from build123d import *

# Parameters (mm, degrees)
SKETCH1_R                      = 5.5
BOSS_EXTRUDE1_DEPTH            = 5
BOSS_EXTRUDE2_DEPTH            = 2
SKETCH4_R                      = 1.4
BOSS_EXTRUDE3_DEPTH            = 7
SKETCH12_W                     = 20
SKETCH12_H                     = 2
CUT_EXTRUDE1_DEPTH             = 10
F_4_2_4_2_DIAMETER_HOLE1_D     = 4.2
F_4_2_4_2_DIAMETER_HOLE1_DEPTH = 20
F_4_2_4_2_DIAMETER_HOLE1_TIP   = 1.2618073
F_5_0_5_DIAMETER_HOLE1_D       = 5
F_5_0_5_DIAMETER_HOLE1_DEPTH   = 5
F_5_0_5_DIAMETER_HOLE1_TIP     = 1.502151548


with BuildPart() as part:
    # Sketch1 → Boss-Extrude1 (new body)
    with BuildSketch(Plane(origin=(0, 111.722415865, 0), x_dir=(1, 0, 0), z_dir=(0, 1, 0))):
        with BuildLine():
            Line((241.95107426, 942.218289838), (411.95107426, 942.218289838))
            ThreePointArc((411.95107426, 942.218289838), (419.022142072, 945.147222026), (421.95107426, 952.218289838))
            Line((421.95107426, 952.218289838), (421.95107426, 1052.218289838))
            ThreePointArc((421.95107426, 1052.218289838), (419.022142072, 1059.28935765), (411.95107426, 1062.218289838))
            Line((411.95107426, 1062.218289838), (241.95107426, 1062.218289838))
            ThreePointArc((241.95107426, 1062.218289838), (234.880006448, 1059.28935765), (231.95107426, 1052.218289838))
            Line((231.95107426, 1052.218289838), (231.95107426, 952.218289838))
            ThreePointArc((231.95107426, 952.218289838), (234.880006448, 945.147222026), (241.95107426, 942.218289838))
        make_face()
        with Locations(Location((241.95107426, 952.218289838, 0), (0, 0, 270))):
            Circle(SKETCH1_R, mode=Mode.SUBTRACT)
        with Locations(Location((411.95107426, 952.218289838, 0), (0, 0, 270))):
            Circle(SKETCH1_R, mode=Mode.SUBTRACT)
        with Locations(Location((411.95107426, 1052.218289838, 0), (0, 0, 270))):
            Circle(SKETCH1_R, mode=Mode.SUBTRACT)
        with Locations(Location((241.95107426, 1052.218289838, 0), (0, 0, 270))):
            Circle(SKETCH1_R, mode=Mode.SUBTRACT)
        with BuildLine():
            Line((249.45107426, 952.218289838), (249.45107426, 944.718289838))
            Line((249.45107426, 944.718289838), (404.45107426, 944.718289838))
            Line((404.45107426, 944.718289838), (404.45107426, 952.218289838))
            ThreePointArc((404.45107426, 952.218289838), (406.647773401, 957.521590697), (411.95107426, 959.718289838))
            Line((411.95107426, 959.718289838), (419.45107426, 959.718289838))
            Line((419.45107426, 959.718289838), (419.45107426, 1044.718289838))
            Line((419.45107426, 1044.718289838), (411.95107426, 1044.718289838))
            ThreePointArc((411.95107426, 1044.718289838), (406.647773401, 1046.914988979), (404.45107426, 1052.218289838))
            Line((404.45107426, 1052.218289838), (404.45107426, 1059.718289838))
            Line((404.45107426, 1059.718289838), (249.45107426, 1059.718289838))
            Line((249.45107426, 1059.718289838), (249.45107426, 1052.218289838))
            ThreePointArc((249.45107426, 1052.218289838), (247.254375119, 1046.914988979), (241.95107426, 1044.718289838))
            Line((241.95107426, 1044.718289838), (234.45107426, 1044.718289838))
            Line((234.45107426, 1044.718289838), (234.45107426, 959.718289838))
            Line((234.45107426, 959.718289838), (241.95107426, 959.718289838))
            ThreePointArc((241.95107426, 959.718289838), (247.254375119, 957.521590697), (249.45107426, 952.218289838))
        make_face(mode=Mode.SUBTRACT)
    extrude(amount=BOSS_EXTRUDE1_DEPTH)

    # Sketch2 → Boss-Extrude2 (add)
    with BuildSketch(Plane(origin=(0, 116.722415865, 0), x_dir=(1, 0, 0), z_dir=(0, 1, 0))):
        with BuildLine():
            Line((231.95107426, 1052.218289838), (231.95107426, 952.218289838))
            ThreePointArc((231.95107426, 952.218289838), (234.880006448, 945.147222026), (241.95107426, 942.218289838))
            Line((241.95107426, 942.218289838), (411.95107426, 942.218289838))
            ThreePointArc((411.95107426, 942.218289838), (419.022142072, 945.147222026), (421.95107426, 952.218289838))
            Line((421.95107426, 952.218289838), (421.95107426, 1052.218289838))
            ThreePointArc((421.95107426, 1052.218289838), (419.022142072, 1059.28935765), (411.95107426, 1062.218289838))
            Line((411.95107426, 1062.218289838), (241.95107426, 1062.218289838))
            ThreePointArc((241.95107426, 1062.218289838), (234.880006448, 1059.28935765), (231.95107426, 1052.218289838))
        make_face()
    extrude(amount=BOSS_EXTRUDE2_DEPTH)

    # Sketch4 → Boss-Extrude3 (add)
    with BuildSketch(Plane(origin=(0, 118.722415865, 0), x_dir=(1, 0, 0), z_dir=(0, 1, 0))):
        with BuildLine():
            Line((375.86522753, 1030.272411662), (375.86522753, 1031.672411662))
            Line((375.86522753, 1031.672411662), (377.26522753, 1031.672411662))
            ThreePointArc((377.26522753, 1031.672411662), (374.875278036, 1032.662361156), (375.86522753, 1030.272411662))
        make_face()
        with BuildLine():
            Line((377.26522753, 1031.672411662), (375.86522753, 1031.672411662))
            Line((375.86522753, 1031.672411662), (375.86522753, 1030.272411662))
            ThreePointArc((375.86522753, 1030.272411662), (376.855177023, 1030.682462168), (377.26522753, 1031.672411662))
        make_face()
        with BuildLine():
            ThreePointArc((377.26522753, 1007.672411662), (376.855177023, 1008.662361156), (375.86522753, 1009.072411662))
            Line((375.86522753, 1009.072411662), (375.86522753, 1007.672411662))
            Line((375.86522753, 1007.672411662), (377.26522753, 1007.672411662))
        make_face()
        with BuildLine():
            Line((375.86522753, 1007.672411662), (375.86522753, 1009.072411662))
            ThreePointArc((375.86522753, 1009.072411662), (374.875278036, 1006.682462168), (377.26522753, 1007.672411662))
            Line((377.26522753, 1007.672411662), (375.86522753, 1007.672411662))
        make_face()
        with Locations(Location((399.86522753, 1031.672411662, 0), (0, 0, 180))):
            Circle(SKETCH4_R)
        with Locations(Location((399.86522753, 1007.672411662, 0), (0, 0, 180))):
            Circle(SKETCH4_R)
    extrude(amount=-BOSS_EXTRUDE3_DEPTH)

    # Sketch12 → Cut-Extrude1 (cut)
    with BuildSketch(Plane(origin=(0, 118.722415865, 0), x_dir=(1, 0, 0), z_dir=(0, 1, 0))):
        with Locations((328.108762335, 982.045276567)):
            Rectangle(SKETCH12_W, SKETCH12_H)
    extrude(amount=-CUT_EXTRUDE1_DEPTH, mode=Mode.SUBTRACT)

    # Ø4.2 (4.2) Diameter Hole1
    with Locations(Plane(origin=(0, 118.722415865, 0), x_dir=(1, 0, 0), z_dir=(0, 1, 0))):
        with Locations((300.990952506, 1024.17077451), (354.990952506, 1024.17077451), (354.990952506, 980.17077451), (300.990952506, 980.17077451)):
            Hole(F_4_2_4_2_DIAMETER_HOLE1_D / 2, depth=F_4_2_4_2_DIAMETER_HOLE1_DEPTH)
            with Locations((0, 0, -(F_4_2_4_2_DIAMETER_HOLE1_DEPTH + F_4_2_4_2_DIAMETER_HOLE1_TIP / 2))):  # 118° drill point
                Cone(0, F_4_2_4_2_DIAMETER_HOLE1_D / 2, F_4_2_4_2_DIAMETER_HOLE1_TIP, mode=Mode.SUBTRACT)

    # Ø5.0 (5) Diameter Hole1
    with Locations(Plane(origin=(0, 118.722415865, 0), x_dir=(1, 0, 0), z_dir=(0, 1, 0))):
        with Locations((241.95107426, 1052.218289838), (411.95107426, 1052.218289838), (411.95107426, 952.218289838), (241.95107426, 952.218289838)):
            Hole(F_5_0_5_DIAMETER_HOLE1_D / 2, depth=F_5_0_5_DIAMETER_HOLE1_DEPTH)
            with Locations((0, 0, -(F_5_0_5_DIAMETER_HOLE1_DEPTH + F_5_0_5_DIAMETER_HOLE1_TIP / 2))):  # 118° drill point
                Cone(0, F_5_0_5_DIAMETER_HOLE1_D / 2, F_5_0_5_DIAMETER_HOLE1_TIP, mode=Mode.SUBTRACT)


solid = part.part
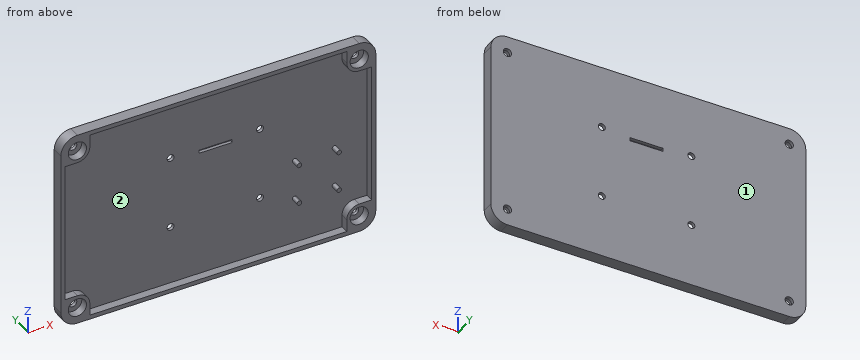
The model under review builds one solid part; all positions refer to its coordinate system, in mm. Face numbers are marked on the shaded views. Coordinates: 2 decimals unless noted, no trailing zeros. Order: outer loops, then holes, each group sorted by start corner. A loop starts at its lowest first (then second) coordinate and runs counter-clockwise, first axis right, second up. Notation, with made-up numbers: (-1, 51) -> (21, 51) arc R18 ccw to (21, 62) -> close; hole circle Ø8 at (-13.75, -37). An arc over 180 degrees is marked (long way). Answer in a Markdown table with one row per item.
(1) The part is to be moulded in two halves that separate along X. For the marked faces 1 and 2, say which applies: +X half, -X half, draft (parallel to the pull), parting line (faces both ways), or undercut.
Answers:
| item | result |
|---|---|
| face 1 | draft |
| face 2 | undercut |
(2) Wall thickness on line 1 along X through (y, z) = (114.25, -1002); line 2 along Z through (x, y) = (295, 114.5); line 3 along X through (y, z) = (116.25, -1007): over which ranges is each line inside the solid? List them lowest first.
Answers:
| item | result |
|---|---|
| line 1 | 231.95 to 234.45, 419.45 to 421.95 |
| line 2 | -1062.22 to -1059.72, -944.72 to -942.22 |
| line 3 | 231.95 to 234.45, 374.64 to 377.09, 398.64 to 401.09, 419.45 to 421.95 |
(3) Insertion check: pin 1 (3.5 mm diameter, centred on x = 239.5, z = -949.5, fed in from -Y); pin 2 (1.5 mm diameter, centred on x = 240, y = 113.5, fed in from +Z). Each pin has a flat end and moves straight along its axis. Give the tip position at first contact, or say it passes through.
Answers:
| item | result |
|---|---|
| pin 1 | y = 116.72 |
| pin 2 | z = -942.29 |
(4) Consider section B-B (z = -998). Write out the cut boundary in (x, y), plus the area to 3 significant figures.
Answers:
| item | result |
|---|---|
| outline | (231.95, 111.72) -> (234.45, 111.72) -> (234.45, 116.72) -> (419.45, 116.72) -> (419.45, 111.72) -> (421.95, 111.72) -> (421.95, 118.72) -> (231.95, 118.72) -> close |
| area | 405 mm² |
(5) Consider section A-A (y = 114.5). State how many separate pieces and enclosed holes the cut face has, plus the area to 3 significant figures.
Answers:
| item | result |
|---|---|
| separate pieces | 5 |
| enclosed holes | 5 |
| area | 1,940 mm² |
(6) Consider section C-C (x = 382). Write out the cut boundary in (y, z).
Answers:
| item | result |
|---|---|
| outline | (111.72, -1062.22) -> (118.72, -1062.22) -> (118.72, -942.22) -> (111.72, -942.22) -> (111.72, -944.72) -> (116.72, -944.72) -> (116.72, -1059.72) -> (111.72, -1059.72) -> close |
